Can you work these out from the model? Positions are in its coordinate system, mm. Round coordinates to 2 decimals unless told otherwise and drop trailing zeros. Loops run counter-clockwise (first coordinate to the right, second up) from the corner with the lowest first, then second, coordinate; pieces in that order, holes last. Notation, with made-up numbers: (69, 63) -> (84, 63) arc R9 cw to (84, 79) -> close; hole circle Ø6 at (-8, 27.25). An arc over 180 degrees is marked (long way). Answer as a JSON object with one key per item and string values.
```python
from build123d import *

# Parameters (mm, degrees)
BOSS_EXTRUDE1_DEPTH             = 76.2
F_1_4_20_START                  = -76.2
F_1_4_20_TAPPED_HOLE2_OUTLINE_R = 2.5527
F_1_4_20_TAPPED_HOLE2_DEPTH     = 76.2


# Read off the part's stored shape, not the designer's step: 1/4-20 Tapped Hole2
with BuildPart() as part:
    # Sketch1 → Boss-Extrude1 (new body)
    with BuildSketch(Plane.XY):
        with BuildLine():
            Line((-4.70551159, -4.549815043), (-3.666174521, -6.349999904))
            Line((-3.666174521, -6.349999904), (-1.587501923, -6.349999904))
            ThreePointArc((-1.587501923, -6.349999904), (-3.85e-07, -4.762498365), (1.587501923, -6.349999904))
            Line((1.587501923, -6.349999904), (3.666173825, -6.349999904))
            Line((3.666173825, -6.349999904), (4.705510929, -4.549815232))
            ThreePointArc((4.705510929, -4.549815232), (4.124445601, -2.381249904), (6.293010929, -1.800184575))
            Line((6.293010929, -1.800184575), (7.332348034, 9.6e-08))
            Line((7.332348034, 9.6e-08), (6.293011178, 1.800184715))
            ThreePointArc((6.293011178, 1.800184715), (4.124445902, 2.381250241), (4.705511428, 4.549815516))
            Line((4.705511428, 4.549815516), (3.666174521, 6.350000222))
            Line((3.666174521, 6.350000222), (1.587498077, 6.350000222))
            ThreePointArc((1.587498077, 6.350000222), (3.85e-07, 4.76250253), (-1.587498077, 6.350000222))
            Line((-1.587498077, 6.350000222), (-3.666173825, 6.350000222))
            Line((-3.666173825, 6.350000222), (-4.705511038, 4.549815614))
            ThreePointArc((-4.705511038, 4.549815614), (-4.124445841, 2.38125025), (-6.293011205, 1.800185053))
            Line((-6.293011205, 1.800185053), (-7.332348419, 4.44e-07))
            Line((-7.332348419, 4.44e-07), (-6.293011423, -1.80018429))
            ThreePointArc((-6.293011423, -1.80018429), (-4.12444613, -2.38124975), (-4.70551159, -4.549815043))
        make_face()
    extrude(amount=-BOSS_EXTRUDE1_DEPTH)

    # 1/4-20 Tapped Hole2 outline → 1/4-20 Tapped Hole2 (cut)
    with BuildSketch(Plane.XY.offset(F_1_4_20_START)):
        Circle(F_1_4_20_TAPPED_HOLE2_OUTLINE_R)
    extrude(amount=F_1_4_20_TAPPED_HOLE2_DEPTH, mode=Mode.SUBTRACT)


solid = part.part
```
Q1. We'd pull the mould along Y, two halves only. Please class faces 1 (the flat face through (4.18, -5.46, -37.57)), 2 (the flat face through (0, -3, -76.2)), 3 (the cylindrical face through (-4.11, 2.41, -37.57)): pulls with the +Y half, pulls with the -Y half, needs draft (parallel to the pull), parting line crosses it, or undercut.
Determined:
{"face 1": "pulls with the -Y half", "face 2": "needs draft", "face 3": "undercut"}
Q2. I'm going to push flat-ended pins straight in: pin 1 (1 mm diameter, centred on y = 2, z = -33.5, fed in from +X); pin 2 (5 mm diameter, centred on x = 4.5, y = -3, fed in from -Z); pin 3 (5 mm diameter, centred on y = 3, z = -64, fed in from -X); pin 4 (5 mm diameter, centred on y = 3, z = -51.5, fed in from +X). Where does each tip first touch, or does it pass through?
Determined:
{"pin 1": "x = 6.47", "pin 2": "z = -76.2", "pin 3": "x = -7.04", "pin 4": "x = 7.04"}
Q3. If I drill on L1, parallel to Y at x = 0, z = -29; L2, parallel to Y at x = -0.25, z = -11.5; L3, parallel to X at y = 5, z = -42, over which ranges is the centre line in solid material (lowest first)? Write a range as [from, to].
Determined:
{"L1": "[-4.76, -2.55], [2.55, 4.76]", "L2": "[-4.78, -2.54], [2.54, 4.78]", "L3": "[-4.45, -0.84], [0.84, 4.45]"}
Q4. I want a section at C-C, the plane y = -5.5. Write out the boundary of the cut face in (x, z), then the cut area to 3 significant figures.
Determined:
{"outline": "(-4.16, -76.2) -> (-1.34, -76.2) -> (-1.34, 0) -> (-4.16, 0) -> close; (1.34, -76.2) -> (4.16, -76.2) -> (4.16, 0) -> (1.34, 0) -> close", "area": "429 mm²"}
Q5. I want a section at A-A, the plane x = 0. Write out the boundary of the cut face in (y, z), then the cut area to 3 significant figures.
Determined:
{"outline": "(-4.76, -76.2) -> (-2.55, -76.2) -> (-2.55, 0) -> (-4.76, 0) -> close; (2.55, -76.2) -> (4.76, -76.2) -> (4.76, 0) -> (2.55, 0) -> close", "area": "337 mm²"}
Q6. I want a section at D-D, the plane y = 3.75. Write out the boundary of the cut face in (x, z), then the cut area to 3 significant figures.
Determined:
{"outline": "(-4.02, -76.2) -> (4.02, -76.2) -> (4.02, 0) -> (-4.02, 0) -> close", "area": "613 mm²"}
